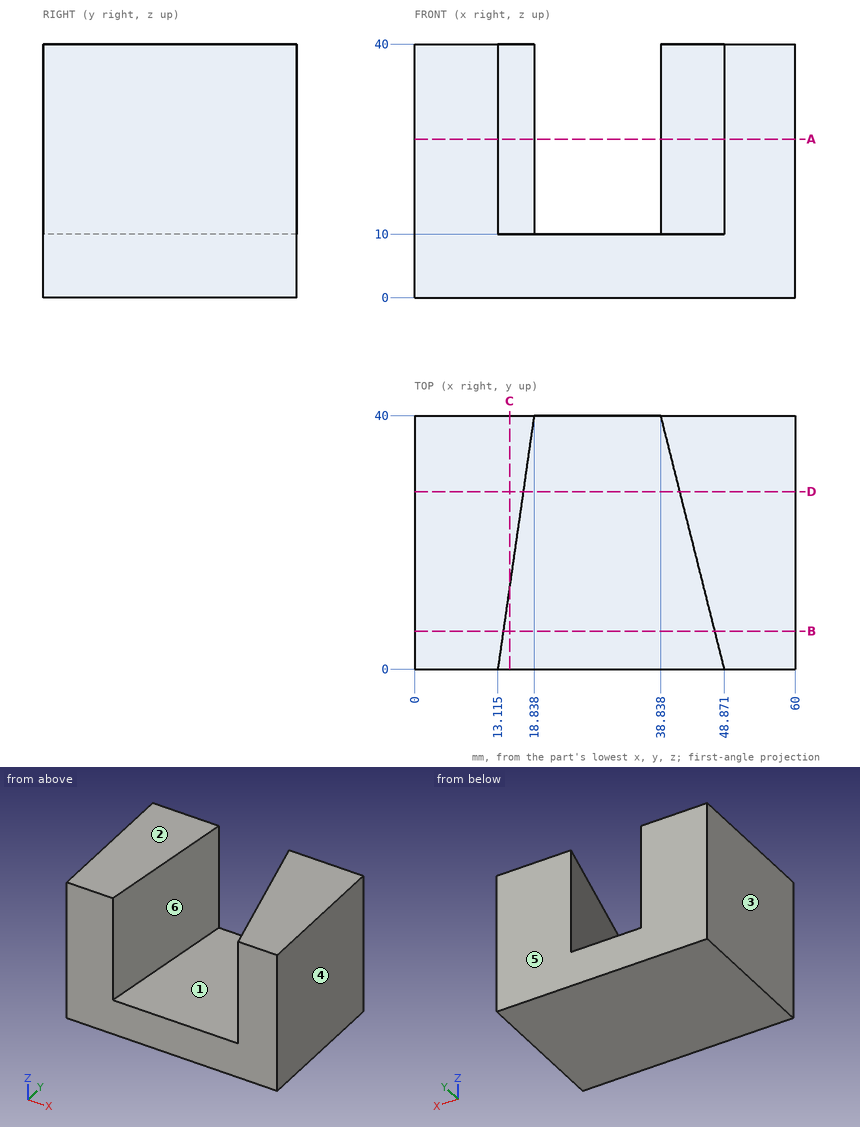
Source: three-view drawing plus pictorial views. Frame: mm from the lowest corner of the part. A direction names the side the tool comes from. Coordinates: 2 decimals unless noted, no trailing zeros. Write each loop counter-clockwise with the first axis right and the second up, starting at its lowest first coordinate (ties: lowest second). Pieces come first, ordered by that corner, then holes. Notation, with made-up numbers: (-20, -24) - (4, -24) arc R16 cw to (4, -16) - close; hole circle Ø10 at (7, 15.5). An arc over 180 degrees is marked (long way). Return JSON: item names as keys, results as strings.
Item 1: Pull-direction query (X, two-part tool) for the marked faces 3, 4, 5 and 6; classes: +X half, -X half, draft (parallel to the pull), parting line (faces both ways), or undercut.
Completed:
{"face 3": "-X half", "face 4": "+X half", "face 5": "draft", "face 6": "undercut"}
Item 2: Section query C-C (x = 15). Output: boundary loops of the cut face in (y, z), and give its area (3 significant figures).
Completed:
{"outline": "(0, 0) - (40, 0) - (40, 40) - (13.18, 40) - (13.18, 10) - (0, 10) - close", "area": "1,200 mm2"}
Item 3: Section query B-B (y = 6). Output: boundary loops of the cut face in (x, z).
Completed:
{"outline": "(0, 0) - (60, 0) - (60, 40) - (47.37, 40) - (47.37, 10) - (13.97, 10) - (13.97, 40) - (0, 40) - close"}
Item 4: Reachability of the marked faces 1 and 2 from +Z, -Z, +X, -X, +Y, -Y: full face, straight path, thin tool, end or side. Return the list, or none.
Completed:
{"face 1": "+Z, -Y", "face 2": "+Z, +X, -X, +Y, -Y"}
Item 5: Section query D-D (y = 28). Output: boundary loops of the cut face in (x, z).
Completed:
{"outline": "(0, 0) - (60, 0) - (60, 40) - (41.85, 40) - (41.85, 10) - (17.12, 10) - (17.12, 40) - (0, 40) - close"}
Item 6: Pin query (flat end, axial travel): pin 1 Ø12 at (x, y) = (28, 31.5) entering from +Z. Return the tip coordinate at first contact, or that it passes through.
Completed:
{"pin 1": "stops at z = 10"}
Item 7: Line query: L1, parallel to Z at x = 29, y = 10; L2, parallel to X at y = 9.5, z = 34 (1 decimal); L3, parallel to X at y = 33, z = 36. Output: solid intervals per line, ascending.
Completed:
{"L1": "z = 0 to 10", "L2": "x = 0 to 14.5, 46.5 to 60", "L3": "x = 0 to 17.84, 40.59 to 60"}
Item 8: Section query A-A (z = 25). Output: boundary loops of the cut face in (x, y) (1 decimal).
Completed:
{"outline": "(0, 0) - (13.1, 0) - (18.8, 40) - (0, 40) - close; (38.8, 40) - (48.9, 0) - (60, 0) - (60, 40) - close"}
